from build123d import *

# Parameters (mm, degrees)
CUT_REVOLVE1_ANGLE = 10
CIRPATTERN1_COUNT  = 20


with BuildPart() as part:
    # Sketch1 → Revolve1 (revolve)
    with BuildSketch(Plane(origin=(0, 0, 0), x_dir=(0, 0, -1), z_dir=(1, 0, 0))):
        with BuildLine():
            Line((45, 0), (42.5, -47.702841719))
            ThreePointArc((42.5, -47.702841719), (50.222540624, -76.742912379), (40, -105))
            Line((40, -105), (42.121320344, -107.121320344))
            ThreePointArc((42.121320344, -107.121320344), (52.934042404, -77.930858803), (45.5, -47.702841719))
            Line((45.5, -47.702841719), (48, 0))
            Line((48, 0), (45, 0))
        make_face()
    revolve(axis=Axis((0, 50.355486862, 0), (0, -1, 0)))

    # Sketch2 → Cut-Revolve1 (revolve, cut)
    with BuildSketch(Plane.XY):
        Polygon((48, 0), (45.5, -47.702841719), (45.374828457, -47.702841719), (47.874828457, 0), align=None)
    cut_revolve1 = revolve(axis=Axis((0, 0, 0), (0, -1, 0)), revolution_arc=CUT_REVOLVE1_ANGLE, mode=Mode.SUBTRACT)

    # CirPattern1: Cut-Revolve1 ×20 about axis
    cirpattern1_axis = Axis((0, 0, 0), (0, 1, 0))
    for i in range(1, CIRPATTERN1_COUNT):
        add(cut_revolve1.rotate(cirpattern1_axis, i * 360 / CIRPATTERN1_COUNT), mode=Mode.SUBTRACT)


solid = part.part
Model file for the job. Use its own axes, mm. A direction names the side the tool comes from. Give positions to 0.01 mm unless a question says otherwise; leave off trailing zeros. Order: outer loops, then holes, each group sorted by start corner. A loop starts at its lowest first (then second) coordinate and runs counter-clockwise, first axis right, second up. Notation, with made-up numbers: (52.5, 50) - (89.5, 50) arc R29 cw to (89.5, 88) - close; hole circle Ø6 at (17.5, 26). An arc over 180 degrees is marked (long way). Return JSON: item names as keys, results as strings.
1) Flat gauge pins, fed straight in: P1, Ø4, axis at y = -73.5, z = -17, coming from the +X side; P2, Ø4, axis at x = 20.5, y = -35, coming from the +Z side; P3, Ø8, axis at x = 9, y = -87.5, coming from the +Z side. Where does each tip first touch, or does it go through?
Geometry says:
{"P1": "x = 50.84", "P2": "z = 42.3", "P3": "z = 51.76"}
2) Cut at A-A, the plane y = -50.5. Give the cut face in (x, z).
Geometry says:
{"outline": "circle Ø94.12 at (0, 0); hole circle Ø88.29 at (0, 0)"}
3) Probe line 1 (X direction, y = -102, z = -1); line 2 (Z direction, x = -7.5, y = -42); line 3 (X direction, y = -89.5, z = -44). List the from-to ranges inside material, lowest first. Write a range as from..to.
Geometry says:
{"line 1": "-45.57..-42.1, 42.1..45.57", "line 2": "-45.05..-42.14, 42.14..45.05", "line 3": "-25.74..-19.17, 19.17..25.74"}
4) Cut at B-B, the plane y = -64. Give the cut face in (x, z), plus the area to 3 significant figures.
Geometry says:
{"outline": "circle Ø103.77 at (0, 0); hole circle Ø98.3 at (0, 0)", "area": "867 mm²"}
5) 3-axis set-ups, long thin cutter, end or side, ignore diameter. For faces 1 (the conical face through (-39.69, -23.52, -24.74)), 2 (the conical face through (-46.65, -23.52, 3.31)), 3 (the conical face through (43, -24, 18)), 4 (the conical face through (30.557, -23.518, -35.239)): which of +Z, -Z, +X, -X, +Y, -Y reach the whole face in a straight line?
Geometry says:
{"face 1": "-Z, -X", "face 2": "+Z, -X", "face 3": "+Z, +X", "face 4": "-Z, +X"}
